Model file for the job. Use its own axes, mm. Face numbers are marked on the shaded views. A direction names the side the tool comes from. Give positions to 0.01 mm unless a question says otherwise; leave off trailing zeros. Write each loop counter-clockwise with the first axis right and the second up, starting at its lowest first coordinate (ties: lowest second). Pieces come first, ordered by that corner, then holes. Notation, with made-up numbers: M 32.5,-37.75 L 82.5,-37.75 A17 cw 82.5,-26.75 Z; hole C -23,-6 d2. An arc over 180 degrees is marked long. Answer as a JSON object with one key per item and string values. Group by question number.
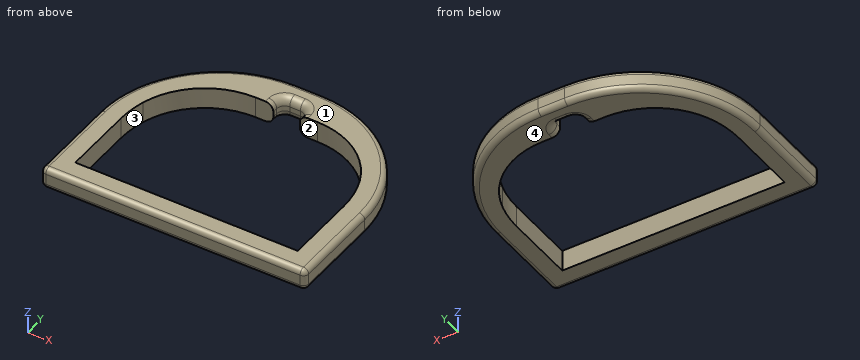
```python
from build123d import *

# Parameters (mm, degrees)
F1_DEPTH = 8
F2_R     = 2
F3_F1_R  = 3
F3_F2_R  = 3


with BuildPart() as f1:
    # F0 (on Top) → F1 (new body)
    with BuildSketch(Plane.XY):
        with BuildLine():
            Line((55, 0), (45, 0))
            ThreePointArc((45, 0), (13.1801948466, -13.1801948466), (0, -45))
            Line((0, -45), (0, -80))
            Line((0, -80), (100, -80))
            Line((100, -80), (100, -45))
            ThreePointArc((100, -45), (86.8198051534, -13.1801948466), (55, 0))
        make_face()
        with BuildLine():
            Line((45, -13), (45, -8))
            Line((45, -8), (55, -8))
            Line((55, -8), (55, -13))
            Line((55, -13), (61.7082039325, -13))
            ThreePointArc((61.7082039325, -13), (79.6366330725, -18.9464882279), (90.4576493575, -34.4285714286))
            ThreePointArc((90.4576493575, -34.4285714286), (91.6123819645, -39.6583254605), (92, -45))
            Line((92, -45), (92, -72))
            Line((92, -72), (8, -72))
            Line((8, -72), (8, -45))
            ThreePointArc((8, -45), (8.3876180355, -39.6583254605), (9.5423506425, -34.4285714286))
            ThreePointArc((9.5423506425, -34.4285714286), (20.3633669275, -18.9464882279), (38.2917960675, -13))
            Line((38.2917960675, -13), (45, -13))
        make_face(mode=Mode.SUBTRACT)
    extrude(amount=F1_DEPTH)

    # F2
    f2_edges = [f1.edges().sort_by_distance(p)[0] for p in [
        (0, -80, 4),
        (100, -80, 4),
        (50, -80, 8),
        (0, -62.5, 8),
        (50, -80, 0),
        (86.819805, -13.180195, 0),
    ]]
    fillet(f2_edges, radius=F2_R)

    # F3: fillet of radius 3 on 4 edges, made by hand

    # F3_f1
    f3_f1_edges = [f1.edges().sort_by_distance(p)[0] for p in [
        (45, -8, 4),
        (55, -8, 4),
    ]]
    fillet(f3_f1_edges, radius=F3_F1_R)

    # F3_f2
    f3_f2_edges = [f1.edges().sort_by_distance(p)[0] for p in [
        (50, -8, 0),
        (50, -8, 8),
        (45.8786796564, -8.8786796564, 8),
        (54.1213203436, -8.8786796564, 8),
        (45.8786796564, -8.8786796564, 0),
        (54.1213203436, -8.8786796564, 0),
    ]]
    fillet(f3_f2_edges, radius=F3_F2_R)


solid = f1.part
```
Q1. Slice it at A-A, the plane y = -52.5. Write the cut outline in (x, z).
Q2. Two-plate mould, pull along X, no slides. Class the marked faces 3 and 4: +X half, -X half, draft (parallel to the pull), parting line (faces both ways), or undercut.
Q3. Wall check: L1, parallel to X at y = -51, z = 2.5; L2, parallel to X at y = -74, z = 6.25; L3, parallel to X at y = -25.5, z = 1.5. Give the ranges that are in metal, low to high.
Q4. 3-axis set-ups, long thin cutter, end or side, ignore diameter. For the marked faces 1 and 2: which of +Z, -Z, +X, -X, +Y, -Y reach the whole face in a straight line?
Q5. Drop flat-ended pins along their axis: P1, Ø4, axis at y = -9, z = 4, coming from the -X side; P2, Ø1, axis at y = -11.5, z = 3.5, coming from the -X side; P3, Ø2, axis at y = -11.5, z = 3.5, coming from the +X side. Give the stop position or say it passes through.
Solved:
{
 "1": {"outline": "M 0,2 A2 ccw 2,0 L 8,0 L 8,8 L 2,8 A2 ccw 0,6 Z; M 92,0 L 98,0 A2 ccw 100,2 L 100,6 A2 ccw 98,8 L 92,8 Z"},
 "2": {"face 3": "undercut", "face 4": "draft"},
 "3": {"L1": "x = 0 to 8, 92 to 100", "L2": "x = 0.02 to 99.98", "L3": "x = 4.51 to 13.92, 86.08 to 95.49"},
 "4": {"face 1": "+Z, +X, -X, +Y, -Y", "face 2": "+Z, -Z"},
 "5": {"P1": "stops at x = 15.52", "P2": "stops at x = 14.41", "P3": "stops at x = 86.12"}
}
